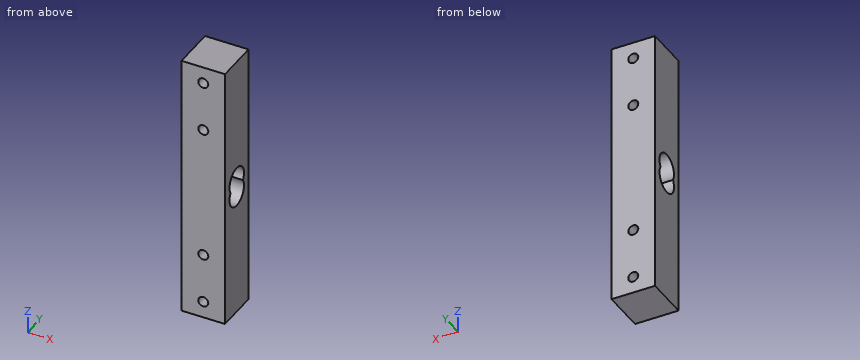
Autodesk Inventor part; units mm, degrees
ref_plane "YZ Plane" through (0, 0, 0) normal (1, 0, 0) x (0, 1, 0)
ref_plane "XZ Plane" through (0, 0, 0) normal (0, 1, 0) x (-1, 0, 0)
ref_plane "XY Plane" through (0, 0, 0) normal (0, 0, 1) x (1, 0, 0)
sketch "Sketch1" plane through (0, 0, 0) normal (0, 1, 0) x (-1, 0, 0)
  line L0 (0, 0) -> (13, 0)
  line L1 (13, 0) -> (13, -80)
  line L2 (13, -80) -> (0, -80)
  line L3 (0, -80) -> (0, 0)
  circle A0 centre (6.5, -60) radius 1.5
  circle A1 centre (6.5, -75) radius 1.5
  circle A2 centre (6.5, -20) radius 1.5
  circle A3 centre (6.5, -5) radius 1.5
  point P0 (6.5, -80)
  point P1 (6.5, 0)
  dimension "d0" = 13
  dimension "d1" = 80
  dimension "d2" = 3
  dimension "d3" = 20
  dimension "d4" = 3
  dimension "d5" = 5
  dimension "d6" = 3
  dimension "d7" = 3
  dimension "d8" = 5
  dimension "d9" = 20
extrude "Extrusion1" add sketch "Sketch1" along normal blind 13
sketch "Sketch2" plane through (0, 0, 0) normal (1, 0, 0) x (0, 0, -1)
  arc A0 (40, 9.9641) -> (40, 3.0359) centre (38, 6.5) ccw
  arc A1 (40, 3.0359) -> (40, 9.9641) centre (42, 6.5) ccw
  line L0 (0, 13) -> (80, 13) construction
  line L1 (80, 0) -> (80, 13) construction
  point P0 (0, 0)
  point P1 (40, 13)
  point P2 (80, 6.5)
  point P3 (80, 6.5)
  dimension "d12" = 8
  dimension "d13" = 8
extrude "Extrusion2" cut sketch "Sketch2" against normal blind 13
properties part number "celda" material "Aluminum 6061"
Here's how the part is built. I have some questions about the finished solid (model axes, mm). Give positions to 0.01 mm unless a question says otherwise; leave off trailing zeros. Order: outer loops, then holes, each group sorted by start corner. A loop starts at its lowest first (then second) coordinate and runs counter-clockwise, first axis right, second up. Notation, with made-up numbers: M 39,87.25 L 53,87.25 A14 ccw 53,95.25 Z; hole C 84,50 d6. An arc over 180 degrees is marked long. Use a Markdown table: item, result. Add a question column.
1. Suppose I cut it at C-C (x = -6.5). List the corners of the cut face in (y, z) for me.
2. Suppose I cut it at B-B (z = -60). List the corners of the cut face in (x, y) for me.
3. I need wall thicknesses on probe 1 along X at (y, z) = (6.25, -75); probe 2 along Y at (x, z) = (-4.75, -42); probe 3 along Z at (x, y) = (-6.5, 5.5). Which ranges of each line are inside material? Lowest first, please. Write a range as from..to.
4. Suppose I cut it at D-D (z = -38). List the corners of the cut face in (x, y) for me, and give its area (3 significant figures).
5. Suppose I cut it at A-A (y = 6.5). List the corners of the cut face in (x, z) for me, and give its area (3 significant figures).
6. For pin 1 Ø5 at (y, z) = (1.5, -19.5) entering from +X; pin 2 Ø1.8 at (x, z) = (-6.5, -20) entering from +Y, each with a flat end and sliding along its axis, tell me the tip position at first contact or that it passes through.
Results list:
| question | item | result |
|---|---|---|
| 1 | outline | M 0,-80 L 13,-80 L 13,-76.5 L 0,-76.5 Z; M 0,-73.5 L 13,-73.5 L 13,-61.5 L 0,-61.5 Z; M 0,-58.5 L 13,-58.5 L 13,-21.5 L 0,-21.5 Z; M 0,-18.5 L 13,-18.5 L 13,-6.5 L 0,-6.5 Z; M 0,-3.5 L 13,-3.5 L 13,0 L 0,0 Z; hole M 3.04,-40 A4 ccw long 9.96,-40 A4 ccw long Z |
| 2 | outline | M -13,0 L -8,0 L -8,13 L -13,13 Z; M -5,0 L 0,0 L 0,13 L -5,13 Z |
| 3 | probe 1 | x = -13..-8, -5..0 |
| 3 | probe 2 | y = 0..2.5, 10.5..13 |
| 3 | probe 3 | z = -80..-76.5, -73.5..-61.5, -58.5..-45.87, -34.13..-21.5, -18.5..-6.5, -3.5..0 |
| 4 | outline | M -13,0 L 0,0 L 0,2.5 L -13,2.5 Z; M -13,10.5 L 0,10.5 L 0,13 L -13,13 Z |
| 4 | area | 65.0 mm² |
| 5 | outline | M -13,-80 L 0,-80 L 0,-46 L -13,-46 Z; M -13,-34 L 0,-34 L 0,0 L -13,0 Z; hole C -6.5,-75 d3; hole C -6.5,-60 d3; hole C -6.5,-20 d3; hole C -6.5,-5 d3 |
| 5 | area | 856 mm² |
| 6 | pin 1 | stops at x = 0 |
| 6 | pin 2 | passes through |
